from build123d import *

# Parameters (mm, degrees)
BOSS_EXTRUDE1_DEPTH = 8
SKETCH2_W           = 7.8
SKETCH2_H           = 7
CUT_EXTRUDE1_DEPTH  = 25.04163056
CHAMFER1_SIZE       = 1
FILLET1_R           = 2


with BuildPart() as part:
    # Sketch1 → Boss-Extrude1 (new body)
    with BuildSketch(Plane(origin=(0, 0, 0), x_dir=(1, 0, 0), z_dir=(0, 1, 0))):
        with BuildLine():
            Line((17, 4.7), (17, 15))
            Line((17, 15), (0, 15))
            Line((0, 15), (0, 0))
            Line((0, 0), (17, 0))
            Line((17, 0), (17, 2.3))
            ThreePointArc((17, 2.3), (15.8, 3.5), (17, 4.7))
        make_face()
    extrude(amount=BOSS_EXTRUDE1_DEPTH)

    # Sketch2 → Cut-Extrude1 (cut, through all)
    with BuildSketch(Plane(origin=(17, 0, 0), x_dir=(0, 0, -1), z_dir=(1, 0, 0))):
        with Locations((11.1, 4.5)):
            Rectangle(SKETCH2_W, SKETCH2_H)
    extrude(amount=-CUT_EXTRUDE1_DEPTH, mode=Mode.SUBTRACT)

    # Chamfer1
    chamfer1_edges = [part.edges().sort_by_distance(p)[0] for p in [
        (15.8, 8, -3.5),
    ]]
    chamfer(chamfer1_edges, length=CHAMFER1_SIZE)

    # Mirror1: part across plane


with BuildPart() as part_1:
    add(part.part)
    add(part.part.mirror(Plane(origin=(17, 8, -4.7), x_dir=(0, 0, 1), z_dir=(-1, 0, 0))))

    # Mirror2: part across plane


with BuildPart() as part_2:
    add(part_1.part)
    add(part_1.part.mirror(Plane(origin=(0, 8, -15), x_dir=(1, 0, 0), z_dir=(0, 0, 1))))

    # Fillet1
    fillet1_edges = [part_2.edges().sort_by_distance(p)[0] for p in [
        (0, 4, 0),
        (34, 4, 0),
        (0, 4, -30),
        (34, 4, -30),
    ]]
    fillet(fillet1_edges, radius=FILLET1_R)


solid = part_2.part
Geometry: final body of the model. Coordinates: model frame, mm. A direction names the side the tool comes from. Give positions to 0.01 mm unless a question says otherwise; leave off trailing zeros. Order: outer loops, then holes, each group sorted by start corner. A loop starts at its lowest first (then second) coordinate and runs counter-clockwise, first axis right, second up. Notation, with made-up numbers: (77, 73.25) -> (113, 73.25) arc R21 cw to (113, 78.25) -> close; hole circle Ø10 at (73.25, 71.5). An arc over 180 degrees is marked (long way). Write each question's results on one line, items separated by ' | '.
1) Cut plane C-C (x = 24). Output: boundary loops of the cut face in (y, z), and give its area (3 significant figures).
Geometry says:
outline: (0, -30) -> (8, -30) -> (8, -22.8) -> (1, -22.8) -> (1, -7.2) -> (8, -7.2) -> (8, 0) -> (0, 0) -> close | area: 131 mm²
2) Draft query along Z for faces 3 (the face through (17, 4, -30)), 4 (the face through (17, 1, -15)), 5 (the face through (17, 4, -22.8)), 6 (the face through (17, 0, -15)). Return one class per face: released by +Z, released by -Z, zero draft, split by the parting line, or undercut.
Geometry says:
face 3: released by -Z | face 4: undercut | face 5: undercut | face 6: zero draft
3) Cut plane B-B (z = -26.5). Output: boundary loops of the cut face in (x, y).
Geometry says:
outline: (0, 0) -> (15.8, 0) -> (15.8, 7) -> (14.8, 8) -> (0, 8) -> close; (18.2, 0) -> (34, 0) -> (34, 8) -> (19.2, 8) -> (18.2, 7) -> close
4) Set-up query: faces 1 (the face through (17, 4, -7.2)), 2 (the face through (0.6, 4.06, -0.57)). Return all of +Z, -Z, +X, -X, +Y, -Y with unobstructed straight access to the full face (end or side cutting, diameter ignored); none if empty.
Geometry says:
face 1: +X, -X, +Y | face 2: +Z, -X, +Y, -Y
5) Cut plane A-A (y = 7.5). Output: boundary loops of the cut face in (x, z), and give its area (3 significant figures).
Geometry says:
outline: (0, -28) arc R2 ccw to (2, -30) -> (32, -30) arc R2 ccw to (34, -28) -> (34, -22.8) -> (0, -22.8) -> close; (0, -7.2) -> (34, -7.2) -> (34, -2) arc R2 ccw to (32, 0) -> (2, 0) arc R2 ccw to (0, -2) -> close; hole circle Ø3.4 at (17, -26.5); hole circle Ø3.4 at (17, -3.5) | area: 468 mm²
6) Cut plane D-D (z = -13). Output: boundary loops of the cut face in (x, y), and give its area (3 significant figures).
Geometry says:
outline: (0, 0) -> (34, 0) -> (34, 1) -> (0, 1) -> close | area: 34.0 mm²
7) First-contact query: pin 1 Ø4.5 at (x, z) = (12.5, -16.5) entering from +Y. Flat tip, straight axial feed; report the tip coordinate or a pass-through.
Geometry says:
pin 1: stops at y = 1
8) Line query: line 1 along Z through (x, y) = (12.5, 5); line 2 along Y through (x, z) = (11, -13.5); line 3 along X through (y, z) = (5, -26.5). Output: solid intervals per line, ascending.
Geometry says:
line 1: z = -30 to -22.8, -7.2 to 0 | line 2: y = 0 to 1 | line 3: x = 0 to 15.8, 18.2 to 34
